```python
from build123d import *

# Parameters (mm, degrees)
F0_W     = 14.976
F0_H     = 20
F1_DEPTH = 2
F3_DEPTH = 10


with BuildPart() as f1:
    # F0 (on Top) → F1 (new body)
    with BuildSketch(Plane.XY):
        with Locations((7.488, 10)):
            Rectangle(F0_W, F0_H)
    extrude(amount=-F1_DEPTH)

    # F2 (on face) → F3 (join)
    with BuildSketch(Plane.XZ):
        with BuildLine():
            Line((7.488, 2), (7.488, 0))
            Line((7.488, 0), (10.488, 0))
            Line((10.488, 0), (10.488, 2.4169947557))
            ThreePointArc((10.488, 2.4169947557), (9.0024210632, 2.1047474172), (7.488, 2))
        make_face()
        with BuildLine():
            Line((4.488, 2.4169947557), (4.488, 0))
            Line((4.488, 0), (7.488, 0))
            Line((7.488, 0), (7.488, 2))
            ThreePointArc((7.488, 2), (5.9735789368, 2.1047474172), (4.488, 2.4169947557))
        make_face()
        with BuildLine():
            Line((4.488, 5), (4.488, 2.4169947557))
            ThreePointArc((4.488, 2.4169947557), (5.9735789368, 2.1047474172), (7.488, 2))
            Line((7.488, 2), (7.488, 5))
            Line((7.488, 5), (4.488, 5))
        make_face()
        with BuildLine():
            Line((7.488, 5), (7.488, 2))
            ThreePointArc((7.488, 2), (9.0024210632, 2.1047474172), (10.488, 2.4169947557))
            Line((10.488, 2.4169947557), (10.488, 5))
            Line((10.488, 5), (7.488, 5))
        make_face()
        with BuildLine():
            ThreePointArc((15.488, 13), (13.1448542495, 7.3431457505), (7.488, 5))
            Line((7.488, 5), (10.488, 5))
            Line((10.488, 5), (10.488, 2.4169947557))
            ThreePointArc((10.488, 2.4169947557), (16.2629643874, 6.3667504193), (18.488, 13))
            ThreePointArc((18.488, 13), (17.4573856574, 17.6488008791), (14.5586637066, 21.4264888743))
            Line((14.5586637066, 21.4264888743), (12.6303008775, 19.128355545))
            ThreePointArc((12.6303008775, 19.128355545), (14.7384622963, 16.3809460939), (15.488, 13))
        make_face()
        with BuildLine():
            ThreePointArc((-3.512, 13), (-1.2869643874, 6.3667504193), (4.488, 2.4169947557))
            Line((4.488, 2.4169947557), (4.488, 5))
            Line((4.488, 5), (7.488, 5))
            ThreePointArc((7.488, 5), (1.8311457505, 7.3431457505), (-0.512, 13))
            Line((-0.512, 13), (-3.512, 13))
        make_face()
        with BuildLine():
            ThreePointArc((0.4173362934, 21.4264888743), (-2.4813856574, 17.6488008791), (-3.512, 13))
            Line((-3.512, 13), (-0.512, 13))
            ThreePointArc((-0.512, 13), (0.2375377037, 16.3809460939), (2.3456991225, 19.128355545))
            Line((2.3456991225, 19.128355545), (0.4173362934, 21.4264888743))
        make_face()
    extrude(amount=-F3_DEPTH)


solid = f1.part
```
The listing builds one solid part. Answer for the finished solid, in the listing's coordinates (mm). A direction names the side the tool comes from. Give positions to 0.01 mm unless a question says otherwise; leave off trailing zeros. Loops run counter-clockwise (first coordinate to the right, second up) from the corner with the lowest first, then second, coordinate; pieces in that order, holes last. Notation, with made-up numbers: (42, 37) - (81, 37) arc R9 cw to (81, 41) - close; hole circle Ø4 at (45, -38). An arc over 180 degrees is marked (long way). Answer as CSV lines item,"result". Start each with the question number.
Item 1: A cutting plane is placed at D-D on z = 10.75. Determine the outline of the cut face in (x, y).
Item 2: For faces 5 (the face through (4.488, 5, 1)), 6 (the face through (14.976, 10, -1)), 7 (the face through (7, 12, 0)), determine the directions among +Z, -Z, +X, -X, +Y, -Y from which every point of the face is accessible in a straight line to the end or side of a thin tool.
Item 3: Each of these flat-tipped pins is pushed along its axis until it touches: pin 1 (2 mm diameter, centred on x = 6.5, z = 3, fed in from -Y); pin 2 (0.7 mm diameter, centred on y = 7, z = 1.5, fed in from -X); pin 3 (1.6 mm diameter, centred on y = 11.5, z = -1.5, fed in from +X); pin 4 (4 mm diameter, centred on x = 1.5, z = 9, fed in from +Y). Where does it stop, or does it pass through?
Item 4: The mould has two halves that part along X. Classify faces 1 (the face through (7, 10, -2)), 2 (the face through (1.395, 4.93, 20.261)), 3 (the face through (0, 10, -1)), 4 (the face through (13.608, 4.93, 20.294)): +X half, -X half, draft (parallel to the pull), parting line (faces both ways), or undercut.
Item 5: A cutting plane is placed at A-A on z = 15. Determine the outline of the cut face in (x, y), then the cut area to 3 significant figures.
Item 6: A cutting plane is placed at C-C on y = 6.25. Determine the outline of the cut face in (x, z), then the cut area to 3 significant figures.
Item 7: Find the intervals of material crossed by line 1 (Y direction, x = 0.75, z = 20.25); line 2 (Z direction, x = 2.75, y = 8.25); line 3 (X direction, y = 3.25, z = 17.5), in increasing order. Write a range as from..to.
Item 8: A cutting plane is placed at B-B on x = 14. Determine the outline of the cut face in (y, z).
Found:
1,outline,"(-3.28, 0) - (-0.19, 0) - (-0.19, 10) - (-3.28, 10) - close; (15.17, 0) - (18.26, 0) - (18.26, 10) - (15.17, 10) - close"
2,face 5,"-X, +Y, -Y"
2,face 6,"-Z, +X, +Y, -Y"
2,face 7,"+Y"
3,pin 1,"stops at y = 0"
3,pin 2,"stops at x = 4.49"
3,pin 3,"stops at x = 14.98"
3,pin 4,"stops at y = 10"
4,face 1,"draft"
4,face 2,"undercut"
4,face 3,"-X half"
4,face 4,"undercut"
5,outline,"(-3.33, 0) - (-0.26, 0) - (-0.26, 10) - (-3.33, 10) - close; (15.23, 0) - (18.3, 0) - (18.3, 10) - (15.23, 10) - close"
5,area,"61.4 mm^2"
6,outline,"(0, -2) - (14.98, -2) - (14.98, 0) - (10.49, 0) - (10.49, 2.42) arc R11 ccw to (14.56, 21.43) - (12.63, 19.13) arc R8 cw (long way) to (2.35, 19.13) - (0.42, 21.43) arc R11 ccw to (4.49, 2.42) - (4.49, 0) - (0, 0) - close"
6,area,"182 mm^2"
7,line 1,"y = 0..10"
7,line 2,"z = -2..0, 3.07..6.55"
7,line 3,"x = -2.55..0.87, 14.1..17.53"
8,outline,"(0, -2) - (20, -2) - (20, 0) - (0, 0) - close; (0, 4.13) - (10, 4.13) - (10, 8.35) - (0, 8.35) - close; (0, 17.65) - (10, 17.65) - (10, 20.76) - (0, 20.76) - close"
